from build123d import *

# Parameters (mm, degrees)
CHAMFER1_SIZE       = 0.5
SKETCH2_R           = 7.5
SKETCH2_R_2         = 5
BOSS_EXTRUDE1_DEPTH = 3


with BuildPart() as part:
    # Sketch1 → Revolve1 (revolve)
    with BuildSketch(Plane.XY):
        Polygon((0, 0), (0, 8), (9.6, 8), (9.6, 5), (17.6, 5), (17.6, 0), align=None)
    revolve(axis=Axis((17.6, 0, 0), (-1, 0, 0)))

    # Chamfer1
    chamfer1_edges = [part.edges().sort_by_distance(p)[0] for p in [
        (0, -8, 0),
    ]]
    chamfer(chamfer1_edges, length=CHAMFER1_SIZE)

    # Sketch2 → Boss-Extrude1 (add)
    with BuildSketch(Plane(origin=(17.6, 0, 0), x_dir=(0, 0, -1), z_dir=(1, 0, 0))):
        with Locations(Location((0, 0, 0), (0, 0, 90))):
            Circle(SKETCH2_R)
        with Locations(Location((0, 0, 0), (0, 0, 90))):
            Circle(SKETCH2_R_2, mode=Mode.SUBTRACT)
    extrude(amount=-BOSS_EXTRUDE1_DEPTH)


solid = part.part
CAD build for the part. Positions are in the model's coordinates, mm. A direction names the side the tool comes from. Coordinates: 2 decimals unless noted, no trailing zeros. Order: outer loops, then holes, each group sorted by start corner. A loop starts at its lowest first (then second) coordinate and runs counter-clockwise, first axis right, second up.
Item 1: Pin check, flat tips, straight feed: pin 1 Ø1 at (x, y) = (7, -2.5) entering from -Z; pin 2 Ø1 at (y, z) = (-5, -5.5) entering from -X; pin 3 Ø4 at (x, z) = (4, -3.5) entering from -Y; pin 4 Ø4 at (x, z) = (12, -2.5) entering from +Y. Stop position of each tip, or through.
Check sheet entries:
pin 1: stops at z = -7.75
pin 2: stops at x = 0
pin 3: stops at y = -7.86
pin 4: stops at y = 4.97
Item 2: Band-saw the part on A-A on z = 0. List the corners of the cut face in (x, y), plus the area to 3 significant figures.
Check sheet entries:
outline: (0, -7.5) - (0.5, -8) - (9.6, -8) - (9.6, -5) - (14.6, -5) - (14.6, -7.5) - (17.6, -7.5) - (17.6, 7.5) - (14.6, 7.5) - (14.6, 5) - (9.6, 5) - (9.6, 8) - (0.5, 8) - (0, 7.5) - close
area: 248 mm2
Item 3: Two-plate mould, pull along X, no slides. Class faces 4 (the face through (5.11, -1.73, 7.81)), 5 (the face through (12.14, -1.08, 4.88)), 6 (the face through (0, 0, 0)): +X half, -X half, draft (parallel to the pull), parting line (faces both ways), or undercut.
Check sheet entries:
face 4: draft
face 5: undercut
face 6: -X half
Item 4: Band-saw the part on C-C on x = 12. List the corners of the cut face in (y, z).
Check sheet entries:
outline: circle Ø10 at (0, 0)
Item 5: 3-axis set-ups, long thin cutter, end or side, ignore diameter. For faces 1 (the face through (17.6, 0, 0)), 2 (the face through (14.6, 2, -5)), 3 (the face through (16.121, -7.493, 0.33)): which of +Z, -Z, +X, -X, +Y, -Y reach the whole face in a straight line?
Check sheet entries:
face 1: +Z, -Z, +X, +Y, -Y
face 2: none
face 3: +X
Item 6: Drill centre lines: L1, parallel to X at y = -4.75, z = -3.75; L2, parallel to Z at x = 16.5, y = 0; L3, parallel to Z at x = 7.5, y = -3.5. Where is each one in solid material? Low to high.
Check sheet entries:
L1: x = 0 to 9.6, 14.6 to 17.6
L2: z = -7.5 to 7.5
L3: z = -7.19 to 7.19
Item 7: Band-saw the part on D-D on x = 3. List the corners of the cut face in (y, z), plus the area to 3 significant figures.
Check sheet entries:
outline: circle Ø16 at (0, 0)
area: 201 mm2
